For this review, take the finished solid that the model builds, in its own axes (mm). Coordinates: 2 decimals unless noted, no trailing zeros. Write each loop counter-clockwise with the first axis right and the second up, starting at its lowest first coordinate (ties: lowest second). Pieces come first, ordered by that corner, then holes. Notation, with made-up numbers: M 74.25,45.5 L 95.25,45.5 A29 ccw 95.25,79.5 Z; hole C 17.5,24.5 d9. An arc over 180 degrees is marked long. One line per question, with ' | ' between items.
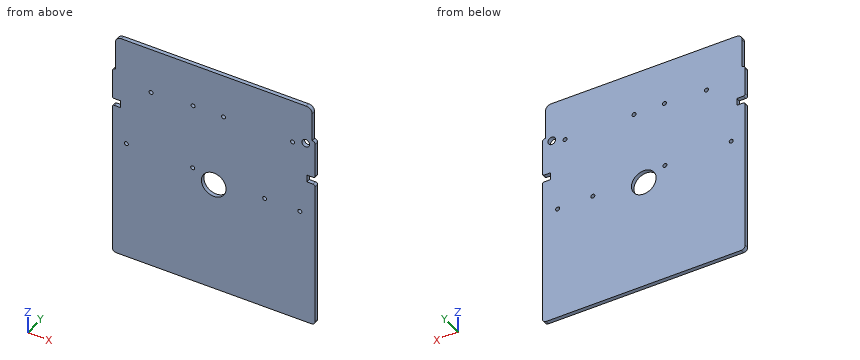
from build123d import *

# Parameters (mm, degrees)
BOSS_EXTRUDE1_DEPTH     = 1
SKETCH2_W               = 2.1
SKETCH2_H               = 1.8
CUT_EXTRUDE1_DEPTH      = 1
CUT_EXTRUDE1_DEPTH_BACK = 2
FILLET1_R               = 0.5
SKETCH3_R               = 0.5
SKETCH3_R_2             = 0.975
CUT_EXTRUDE2_DEPTH      = 1
CUT_EXTRUDE2_DEPTH_BACK = 2


with BuildPart() as part:
    # Sketch1 → Boss-Extrude1 (new body)
    with BuildSketch(Plane(origin=(0, 0, 0), x_dir=(1, 0, 0), z_dir=(0, 1, 0))):
        with BuildLine():
            Line((0, -1), (0, -21.45))
            ThreePointArc((0, -21.45), (0.219669914, -21.980330086), (0.75, -22.2))
            Line((0.75, -22.2), (0.75, -29.3))
            ThreePointArc((0.75, -29.3), (1.189339828, -30.360660172), (2.25, -30.8))
            Line((2.25, -30.8), (48.75, -30.8))
            ThreePointArc((48.75, -30.8), (49.810660172, -30.360660172), (50.25, -29.3))
            Line((50.25, -29.3), (50.25, -22.2))
            ThreePointArc((50.25, -22.2), (50.780330086, -21.980330086), (51, -21.45))
            Line((51, -21.45), (51, -1))
            Line((51, -1), (51, 25.5))
            ThreePointArc((51, 25.5), (50.707106781, 26.207106781), (50, 26.5))
            Line((50, 26.5), (1, 26.5))
            ThreePointArc((1, 26.5), (0.292893219, 26.207106781), (0, 25.5))
            Line((0, 25.5), (0, -1))
        make_face()
    extrude(amount=BOSS_EXTRUDE1_DEPTH)

    # Sketch2 → Cut-Extrude1 (cut, two sides)
    with BuildSketch(Plane(origin=(0, 1, 0), x_dir=(1, 0, 0), z_dir=(0, 1, 0))) as cut_extrude1_sk:
        with Locations((1.05, -13.35)):
            Rectangle(SKETCH2_W, SKETCH2_H)
        with BuildLine():
            ThreePointArc((22.4, -1), (25.5, -4.1), (28.6, -1))
            ThreePointArc((28.6, -1), (25.5, 2.1), (22.4, -1))
        make_face()
        with Locations((49.95, -11.65)):
            Rectangle(SKETCH2_W, SKETCH2_H)
    extrude(amount=CUT_EXTRUDE1_DEPTH, mode=Mode.SUBTRACT)
    extrude(cut_extrude1_sk.sketch, amount=-CUT_EXTRUDE1_DEPTH_BACK, mode=Mode.SUBTRACT)

    # Fillet1
    fillet1_edges = [part.edges().sort_by_distance(p)[0] for p in [
        (0, 0.5, 14.25),
        (0, 0.5, 12.45),
        (51, 0.5, 10.75),
        (51, 0.5, 12.55),
    ]]
    fillet(fillet1_edges, radius=FILLET1_R)

    # Sketch3 → Cut-Extrude2 (cut, two sides)
    with BuildSketch(Plane(origin=(0, 1, 0), x_dir=(1, 0, 0), z_dir=(0, 1, 0))) as cut_extrude2_sk:
        with Locations((3.52, -3.45)):
            Circle(SKETCH3_R)
        with Locations((20.2, -3.45)):
            Circle(SKETCH3_R)
        with Locations((38.3, -2.25)):
            Circle(SKETCH3_R)
        with Locations((47.14, -2.25)):
            Circle(SKETCH3_R)
        with Locations((48.627, -20.91)):
            Circle(SKETCH3_R_2)
        with Locations((45.29, -19.95)):
            Circle(SKETCH3_R)
        with Locations((27.94, -19.95)):
            Circle(SKETCH3_R)
        with Locations((20.29, -19.95)):
            Circle(SKETCH3_R)
        with Locations((9.75, -19.43)):
            Circle(SKETCH3_R)
    extrude(amount=CUT_EXTRUDE2_DEPTH, mode=Mode.SUBTRACT)
    extrude(cut_extrude2_sk.sketch, amount=-CUT_EXTRUDE2_DEPTH_BACK, mode=Mode.SUBTRACT)


solid = part.part
1) We need section C-C on z = 24. State the section outline as (x, y) points.
Responses:
outline: M 0.75,0 L 50.25,0 L 50.25,1 L 0.75,1 Z
2) To check wall thickness, follow line 1 along Z through (x, y) = (20.29, 0.75); line 2 along Z through (x, y) = (3.52, 0.5); line 3 along Z through (x, y) = (47.14, 0.75). State the ranges of each line that lie inside material, in increasing order. Write a range as [from, to].
Responses:
line 1: [-26.5, 2.96], [3.94, 19.45], [20.45, 30.8] | line 2: [-26.5, 2.95], [3.95, 30.8] | line 3: [-26.5, 1.75], [2.75, 30.8]
3) We need section A-A on y = 0.6. State how many separate pieces and enclosed holes the cut face has, then the cut area to 3 significant figures.
Responses:
separate pieces: 1 | enclosed holes: 10 | area: 2,860 mm^2
4) Insertion check: pin 1 Ø5.5 at (x, z) = (25.5, 1) entering from +Y; pin 2 Ø0.5 at (y, z) = (0.5, 13.5) entering from -X. Each pin has a flat end and moves straight along its axis. Give the tip position at first contact, or say it passes through.
Responses:
pin 1: through | pin 2: x = 2.1
5) We need section B-B on z = 1. State the section outline as (x, y) points, then the cut area to 3 significant figures.
Responses:
outline: M 0,0 L 22.4,0 L 22.4,1 L 0,1 Z; M 28.6,0 L 51,0 L 51,1 L 28.6,1 Z | area: 44.8 mm^2
